The model under review builds one solid part; all positions refer to its coordinate system, in mm. A direction names the side the tool comes from. Give positions to 0.01 mm unless a question says otherwise; leave off trailing zeros. Loops run counter-clockwise (first coordinate to the right, second up) from the corner with the lowest first, then second, coordinate; pieces in that order, holes last. Notation, with made-up numbers: (-7.5, 30) -> (27.5, 30) arc R10 cw to (27.5, 44) -> close; hole circle Ø6 at (-30, 34). An arc over 180 degrees is marked (long way). Write each question's results on one line, items separated by ' | '. Start each with the question number.
Q1. Mouldability with a two-part tool opening along X and no side actions: class faces 5 (the face through (-24.56, 1, -0.32)), 6 (the face through (-27, -1, 0.375)), 7 (the face through (-26.2, 0, 0)), 8 (the face through (0, 0, 0)) as released by +X, released by -X, zero draft, split by the parting line, or undercut.
Q2. We need section D-D (z = 2.1). Write out the cut boundary in (x, y).
Q3. Machinability: for faces 1 (the face through (-25, -1.21, -0.04)), 2 (the face through (-25.4, -2.8, -0.1)), 3 (the face through (-27, -0.375, 1)), 4 (the face through (-12.22, -1.5, -0.07)), which of the approach directions +Z, -Z, +X, -X, +Y, -Y give a long, thin tool a straight path to every point of the face, cutting with its end or side? Answer none if there is none.
Q4. We need section A-A (z = 0). Write out the cut boundary in (x, y).
Q5. Insertion check: pin 1 Ø2 at (x, z) = (-6.5, 0) entering from -Y; pin 2 Ø1.5 at (x, y) = (-10.5, 1.5) entering from -Z; pin 3 Ø0.9 at (x, z) = (-27, 1) entering from -Y. Each pin has a flat end and moves straight along its axis. Give the tip position at first contact, or say it passes through.
Q6. We need section C-C (x = -11.75). Write out the cut boundary in (y, z), plus the area to 3 significant figures.
Q7. Wall thickness on L1, parallel to X at y = 0.15, z = 1.3; L2, parallel to X at y = 0.65, z = -1.25; L3, parallel to Z at x = -12.5, y = -0.1: over which ranges is each line inside the solid? List them lowest first. Write a range as [from, to].
from build123d import *

# Parameters (mm, degrees)
CUT_EXTRUDE_5_DEPTH = 1.2


with BuildPart() as part:
    # 草图2 → 旋转1 (revolve)
    with BuildSketch(Plane.XY):
        with BuildLine():
            Line((0, 0), (0, 1.5))
            Line((0, 1.5), (-24.1, 1.5))
            Line((-24.1, 1.5), (-24.1, 1.05))
            Line((-24.1, 1.05), (-25, 1.05))
            Line((-25, 1.05), (-25, 2.8))
            Line((-25, 2.8), (-25.8, 2.8))
            ThreePointArc((-25.8, 2.8), (-26.971790212, 1.61245155), (-27.4, 0))
            Line((-27.4, 0), (0, 0))
        make_face()
    revolve(axis=Axis((0, 0, 0), (-1, 0, 0)))

    # 草图3 → 切除-拉伸5 (cut)
    with BuildSketch(Plane(origin=(-27.4, 0, 0), x_dir=(0, 0, -1), z_dir=(1, 0, 0))):
        with BuildLine():
            Line((0.375, 1.8), (-0.375, 1.8))
            Line((-0.375, 1.8), (-0.375, 0.675))
            ThreePointArc((-0.375, 0.675), (-0.462867966, 0.462867966), (-0.675, 0.375))
            Line((-0.675, 0.375), (-1.8, 0.375))
            Line((-1.8, 0.375), (-1.8, -0.375))
            Line((-1.8, -0.375), (-0.675, -0.375))
            ThreePointArc((-0.675, -0.375), (-0.462867966, -0.462867966), (-0.375, -0.675))
            Line((-0.375, -0.675), (-0.375, -1.8))
            Line((-0.375, -1.8), (0.375, -1.8))
            Line((0.375, -1.8), (0.375, -0.675))
            ThreePointArc((0.375, -0.675), (0.462867966, -0.462867966), (0.675, -0.375))
            Line((0.675, -0.375), (1.8, -0.375))
            Line((1.8, -0.375), (1.8, 0.375))
            Line((1.8, 0.375), (0.675, 0.375))
            ThreePointArc((0.675, 0.375), (0.462867966, 0.462867966), (0.375, 0.675))
            Line((0.375, 0.675), (0.375, 1.8))
        make_face()
    extrude(amount=CUT_EXTRUDE_5_DEPTH, mode=Mode.SUBTRACT)


solid = part.part
Output:
1) face 5: undercut | face 6: zero draft | face 7: released by -X | face 8: released by +X
2) outline: (-25.8, -1.85) -> (-25, -1.85) -> (-25, 1.85) -> (-25.8, 1.85) arc R2.48 ccw to start
3) face 1: none | face 2: +X, -X | face 3: -X | face 4: +X
4) outline: (-26.86, -1.8) arc R3.25 ccw to (-25.8, -2.8) -> (-25, -2.8) -> (-25, -1.05) -> (-24.1, -1.05) -> (-24.1, -1.5) -> (0, -1.5) -> (0, 1.5) -> (-24.1, 1.5) -> (-24.1, 1.05) -> (-25, 1.05) -> (-25, 2.8) -> (-25.8, 2.8) arc R3.25 ccw to (-26.86, 1.8) -> (-26.2, 1.8) -> (-26.2, -1.8) -> close
5) pin 1: y = -1.5 | pin 2: z = -1.3 | pin 3: y = -1.99
6) outline: circle Ø3 at (0, 0) | area: 7.07 mm2
7) L1: [-26.2, -25], [-24.1, 0] | L2: [-27.08, -25], [-24.1, 0] | L3: [-1.5, 1.5]
